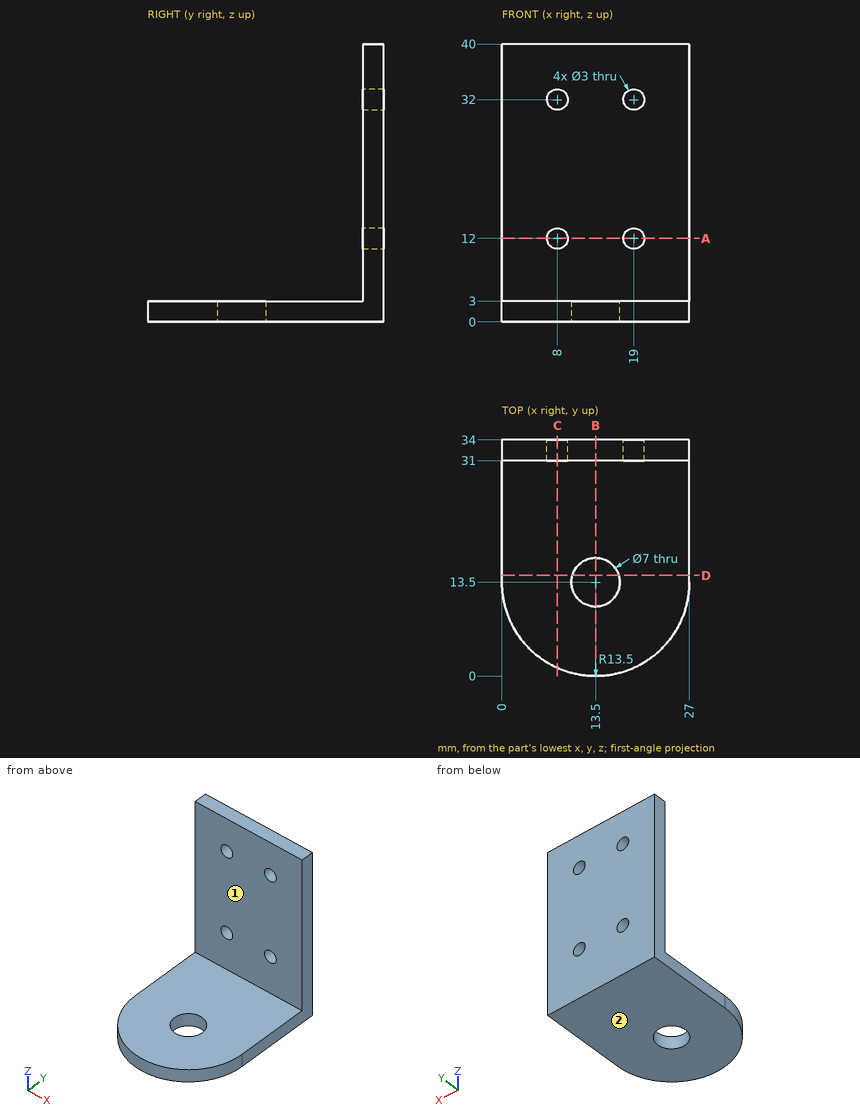
Geometry check sheet. Reference: drawing and pictorial views, mm from the part's lowest x, y, z. A direction names the side the tool comes from. Coordinates: 2 decimals unless noted, no trailing zeros. Order: outer loops, then holes, each group sorted by start corner. A loop starts at its lowest first (then second) coordinate and runs counter-clockwise, first axis right, second up. Notation, with made-up numbers: (77, 78) - (118, 78) arc R9 ccw to (118, 94) - close; hole circle Ø10 at (87.5, -27). An arc over 180 degrees is marked (long way). One line per item, written item: value.
(1) Sectioned sample at A-A (z = 12). Enter the section's corners in (x, y), and give its area (3 significant figures).
Data:
outline: (0, 31) - (6.5, 31) - (6.5, 34) - (0, 34) - close; (9.5, 31) - (17.5, 31) - (17.5, 34) - (9.5, 34) - close; (20.5, 31) - (27, 31) - (27, 34) - (20.5, 34) - close
area: 63.0 mm^2
(2) Access from +Z, -Z, +X, -X, +Y, -Y to the whole of each face (thin tool, end or side, straight path). Record for the marked faces 1 and 2.
Data:
face 1: +Z, +X, -X, -Y
face 2: -Z, +X, -X, +Y, -Y
(3) Sectioned sample at C-C (x = 8). Enter the section's corners in (y, z).
Data:
outline: (1.17, 0) - (34, 0) - (34, 10.5) - (31, 10.5) - (31, 3) - (1.17, 3) - close; (31, 13.5) - (34, 13.5) - (34, 30.5) - (31, 30.5) - close; (31, 33.5) - (34, 33.5) - (34, 40) - (31, 40) - close
(4) Sectioned sample at D-D (y = 14.5). Enter the section's corners in (x, z), and give its area (3 significant figures).
Data:
outline: (0, 0) - (10.15, 0) - (10.15, 3) - (0, 3) - close; (16.85, 0) - (27, 0) - (27, 3) - (16.85, 3) - close
area: 60.9 mm^2
(5) Depth check by flat-ended pin: pin 1 Ø6 at (x, y) = (10.5, 4.5) entering from -Z; pin 2 Ø5 at (x, y) = (16.5, 10) entering from +Z; pin 3 Ø5 at (x, z) = (17.5, 33) entering from -Y. Enter the tip coordinate at first touch or a pass-through.
Data:
pin 1: stops at z = 0
pin 2: stops at z = 3
pin 3: stops at y = 31
(6) Sectioned sample at B-B (x = 13.5). Enter the section's corners in (y, z).
Data:
outline: (0, 0) - (10, 0) - (10, 3) - (0, 3) - close; (17, 0) - (34, 0) - (34, 40) - (31, 40) - (31, 3) - (17, 3) - close
(7) Thickness scan on probe 1 along X at (y, z) = (32, 12); probe 2 along Z at (x, y) = (8, 32.4); probe 3 along X at (y, z) = (13.5, 1.7). Record the ranges inside material, lowest first. Write a range as from..to.
Data:
probe 1: x = 0..6.5, 9.5..17.5, 20.5..27
probe 2: z = 0..10.5, 13.5..30.5, 33.5..40
probe 3: x = 0..10, 17..27
